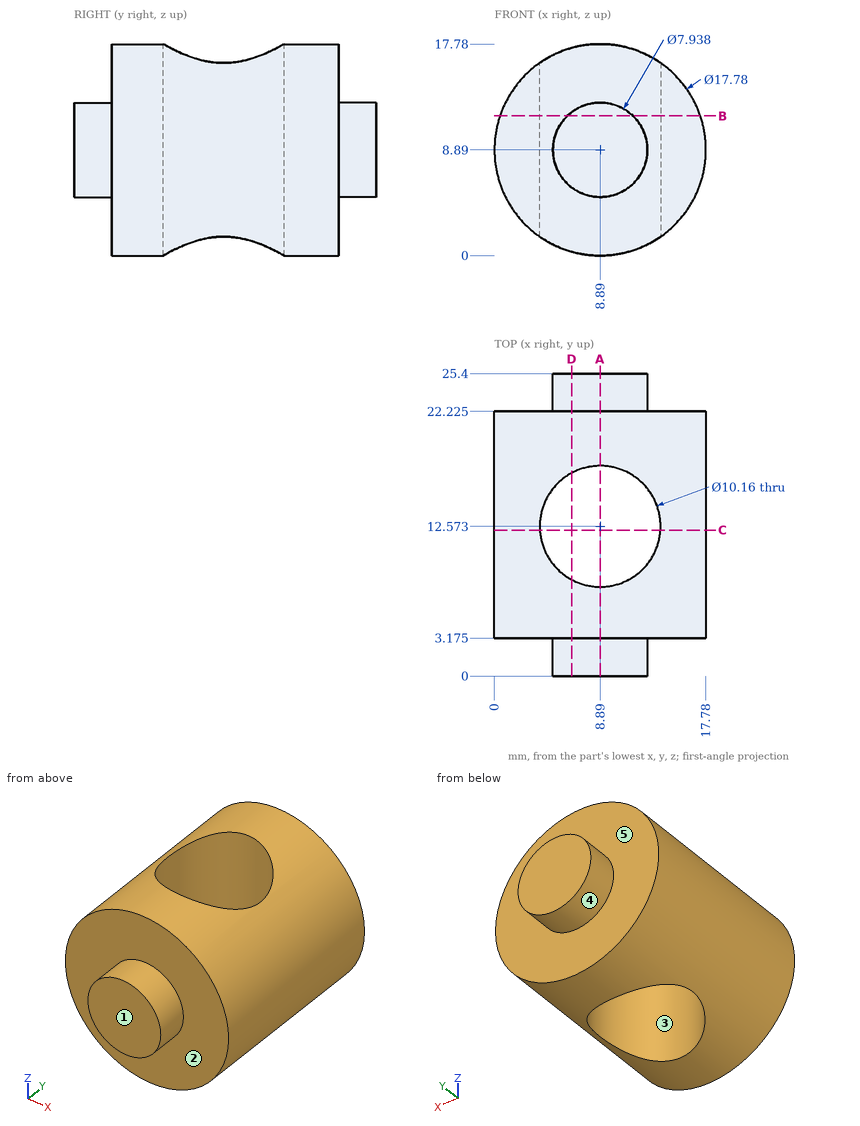
Answer from the drawing. Dimensions are ordinates in mm from the lowest x, y and z of the part. A direction names the side the tool comes from. Give positions to 0.01 mm unless a question says otherwise; leave off trailing zeros. Write each loop counter-clockwise with the first axis right and the second up, starting at its lowest first coordinate (ties: lowest second). Pieces come first, ordered by that corner, then holes.
1) Given P1, Ø4, axis at y = 19, z = 14.5, coming from the -X side (1 decimal); P2, Ø4, axis at x = 5, y = 4, coming from the -Z side; P3, Ø2, axis at x = 5, z = 7, coming from the -Y side; P4, Ø5, axis at y = 17, z = 6, coming from the -X side, each flat-ended and moving along its own axis, determine where each tip first touches the part or whether it passes through.
2) Section D-D (x = 6.5) is taken. Write down the section's boundary in (y, z) (1 decimal).
3) Find the intervals of material crossed by L1, parallel to Y at x = 8.89, z = 10.75; L2, parallel to X at y = 15.5, z = 5 (1 decimal); L3, parallel to X at y = 13.5, z = 8.25 (1 decimal), in increasing order.
4) Section B-B (z = 11.75) is taken. Write down the section's boundary in (x, y) (1 decimal).
5) Section C-C (y = 12.25) is taken. Write down the section's boundary in (x, z).
6) A tool of negligible diameter and unlimited length cuts with its end or side. For the marked faces 1 and 2, from which of +Z, -Z, +X, -X, +Y, -Y can it reach the whole face along a straight path? Write none if from no direction.
7) Section A-A (x = 8.89) is taken. Write down the section's boundary in (y, z) (1 decimal).
8) For a pull along Y with two mould halves and no side action, classify the marked faces 3, 4 and 5 as pulls with the +Y half, pulls with the -Y half, needs draft (parallel to the pull), parting line crosses it, or undercut.
Response:
1. P1: stops at x = 0.8
1. P2: stops at z = 0.2
1. P3: stops at y = 0
1. P4: stops at x = 0.01
2. outline: (0, 5.7) - (3.2, 5.7) - (3.2, 0.3) - (8.1, 0.3) - (8.1, 17.5) - (3.2, 17.5) - (3.2, 12.1) - (0, 12.1) - close; (17.1, 0.3) - (22.2, 0.3) - (22.2, 5.7) - (25.4, 5.7) - (25.4, 12.1) - (22.2, 12.1) - (22.2, 17.5) - (17.1, 17.5) - close
3. L1: y = 0 to 7.49, 17.65 to 25.4
3. L2: x = 0.9 to 4.7, 13 to 16.9
3. L3: x = 0 to 3.9, 13.9 to 17.8
4. outline: (0.5, 3.2) - (6.1, 3.2) - (6.1, 0) - (11.6, 0) - (11.6, 3.2) - (17.3, 3.2) - (17.3, 22.2) - (11.6, 22.2) - (11.6, 25.4) - (6.1, 25.4) - (6.1, 22.2) - (0.5, 22.2) - close; hole circle Ø10.2 at (8.9, 12.6)
5. outline: (3.82, 1.59) - (3.82, 16.19) arc R8.89 ccw to start; (13.96, 1.59) arc R8.89 ccw to (13.96, 16.19) - close
6. face 1: +Z, -Z, +X, -X, -Y
6. face 2: -Y
7. outline: (0, 4.9) - (3.2, 4.9) - (3.2, 0) - (7.5, 0) - (7.5, 17.8) - (3.2, 17.8) - (3.2, 12.9) - (0, 12.9) - close; (17.7, 0) - (22.2, 0) - (22.2, 4.9) - (25.4, 4.9) - (25.4, 12.9) - (22.2, 12.9) - (22.2, 17.8) - (17.7, 17.8) - close
8. face 3: undercut
8. face 4: needs draft
8. face 5: pulls with the +Y half
